Model file for the job. Use its own axes, mm. A direction names the side the tool comes from. Coordinates: 2 decimals unless noted, no trailing zeros. Order: outer loops, then holes, each group sorted by start corner. A loop starts at its lowest first (then second) coordinate and runs counter-clockwise, first axis right, second up. Notation, with made-up numbers: M -24,-36.5 L 30,-36.5 A11 ccw 30,-15.5 Z; hole C -12.75,-25 d5. An arc over 180 degrees is marked long. Return JSON: item names as keys, results as strings.
```python
from build123d import *

# Parameters (mm, degrees)
F0_R     = 22.225
F1_DEPTH = 457.2
F2_W     = 25.4
F2_H     = 63.5
F2_R     = 9.525
F3_DEPTH = 9.525
F4_R     = 7.62


with BuildPart() as f1:
    # F0 (on Top) → F1 (new body)
    with BuildSketch(Plane.XY):
        Circle(F0_R)
    extrude(amount=-F1_DEPTH)

    # F2 (on Front) → F3 (join, symmetric)
    with BuildSketch(Plane.XZ):
        Rectangle(F2_W, F2_H)
        with Locations((0, 17.4507647753)):
            Circle(F2_R, mode=Mode.SUBTRACT)
    extrude(amount=F3_DEPTH, both=True)

    # F4
    f4_edges = [f1.edges().sort_by_distance(p)[0] for p in [
        (12.7, 0, 31.75),
        (-12.7, 0, 31.75),
    ]]
    fillet(f4_edges, radius=F4_R)


solid = f1.part
```
Item 1: Saw through at A-A (x = 0). Write the cut outline in (y, z) (3 decimals), and give its area (3 significant figures).
Check result:
{"outline": "M -22.225,-457.2 L 22.225,-457.2 L 22.225,0 L 9.525,0 L 9.525,7.926 L -9.525,7.926 L -9.525,0 L -22.225,0 Z; M -9.525,26.976 L 9.525,26.976 L 9.525,31.75 L -9.525,31.75 Z", "area": "20,600 mm2"}
Item 2: Wall check: line 1 (Z direction, x = -1, y = 6); line 2 (Z direction, x = 0, y = 3.75); line 3 (X direction, y = 2, z = -152). Give the ranges that are in metal, low to high.
Check result:
{"line 1": "z = -457.2 to 7.98, 26.92 to 31.75", "line 2": "z = -457.2 to 7.93, 26.98 to 31.75", "line 3": "x = -22.13 to 22.13"}
Item 3: 3-axis set-ups, long thin cutter, end or side, ignore diameter. For faces 4 (the flat face through (5, -9.525, 9)), 5 (the flat face through (0, 0, 31.75)), 6 (the flat face through (-12.7, 0, 12)), 7 (the flat face through (0, 0, -457.2)), 8 (the flat face through (12.7, 0, 12)): which of +Z, -Z, +X, -X, +Y, -Y reach the whole face in a straight line?
Check result:
{"face 4": "+Z, +X, -X, -Y", "face 5": "+Z, +X, -X, +Y, -Y", "face 6": "+Z, -X, +Y, -Y", "face 7": "-Z, +X, -X, +Y, -Y", "face 8": "+Z, +X, +Y, -Y"}
Item 4: Pull direction Z, two halves, no side cores. Call faces 1 (the cylindrical face through (-1.2, 0.1, 26.9)), 2 (the flat face through (5, 9.525, 9)), 3 (the cylindrical face through (-10.527, 0.133, 29.459)): +Z half, -Z half, draft (parallel to the pull), parting line (faces both ways), or undercut.
Check result:
{"face 1": "undercut", "face 2": "draft", "face 3": "+Z half"}
Item 5: Saw through at C-C (z = -299.5). Write the cut outline in (x, y) (3 decimals), and give its area (3 significant figures).
Check result:
{"outline": "C 0,0 d44.45", "area": "1,550 mm2"}
Item 6: Drop flat-ended pins along their axis: pin 1 Ø4 at (y, z) = (-13.5, -264) entering from +X; pin 2 Ø2 at (x, y) = (8.5, 16) entering from +Z; pin 3 Ø7.5 at (x, z) = (-3, 23) entering from +Y (3 decimals). Give the stop position or say it passes through.
Check result:
{"pin 1": "stops at x = 19.02", "pin 2": "stops at z = 0", "pin 3": "stops at y = 9.525"}
Item 7: Saw through at B-B (y = -4). Write the cut outline in (x, z) (3 decimals).
Check result:
{"outline": "M -21.862,-457.2 L 21.862,-457.2 L 21.862,0 L 12.7,0 L 12.7,24.13 A7.62 ccw 5.08,31.75 L -5.08,31.75 A7.62 ccw -12.7,24.13 L -12.7,0 L -21.862,0 Z; hole C 0,17.451 d19.05"}
